from build123d import *

# Parameters (mm, degrees)
F0_W          = 105.2140146494
F0_H          = 74.0064755082
F0_R          = 22.3889711498
F1_DEPTH      = 22.86
F2_DEPTH      = 59.944
F3_DEPTH      = 25.4
F3_FACE_R     = 22.3889711498
F4_DEPTH      = 25.4
F4_TAPER      = -3
F5_DEPTH      = 25.4
F5_DEPTH_BACK = 25.4
F5_FACE_R     = 22.3889711498
F6_DEPTH      = 25.4
F6_TAPER      = -15
F7_DEPTH      = 59.182
F9_DEPTH      = 33.274


with BuildPart() as f1:
    # F0 (on Top) → F1 (new body)
    with BuildSketch(Plane.XY):
        Rectangle(F0_W, F0_H)
        Circle(F0_R, mode=Mode.SUBTRACT)
        Circle(F0_R)
    extrude(amount=F1_DEPTH)

    # F0 (on Top) → F2 (join)
    with BuildSketch(Plane.XY):
        Circle(F0_R)
    extrude(amount=F2_DEPTH)

    # F3 (cut): a face of the model
    f3_faces = [f1.faces().sort_by_distance(p)[0] for p in [
        (0, 0, 59.944),
    ]]
    extrude(f3_faces, amount=-F3_DEPTH, mode=Mode.SUBTRACT)

    # F3_face (on face) → F4 (join)
    with BuildSketch(Plane.XY.offset(34.544)):
        Circle(F3_FACE_R)
    extrude(amount=F4_DEPTH, taper=F4_TAPER)

    # F5 (cut, two sides): a face of the model
    f5_faces = [f1.faces().sort_by_distance(p)[0] for p in [
        (0, 0, 59.944),
    ]]
    extrude(f5_faces, amount=-F5_DEPTH, mode=Mode.SUBTRACT)
    extrude(f5_faces, amount=F5_DEPTH_BACK, mode=Mode.SUBTRACT)

    # F5_face (on face) → F6 (cut)
    with BuildSketch(Plane.XY.offset(34.544)):
        Circle(F5_FACE_R)
    extrude(amount=-F6_DEPTH, taper=F6_TAPER, mode=Mode.SUBTRACT)

    # F7 (add): a face of the model
    f7_faces = [f1.faces().sort_by_distance(p)[0] for p in [
        (0, 0, 9.144),
    ]]
    extrude(f7_faces, amount=F7_DEPTH)

    # F8 (on Front) → F9 (cut, symmetric)
    with BuildSketch(Plane.XZ):
        Polygon((-21.8193475157, 85.7371985912), (-29.5202936977, 68.7951147556), (38.5047309101, 34.6542596817), (50.8262440562, 89.5876735449), align=None)
    extrude(amount=F9_DEPTH, both=True, mode=Mode.SUBTRACT)


solid = f1.part
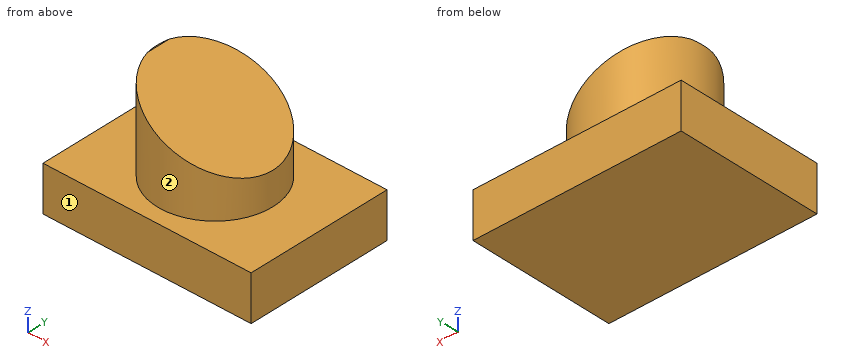
Geometry: final body of the model. Coordinates: model frame, mm. Face numbers are marked on the shaded views. A direction names the side the tool comes from. Coordinates: 2 decimals unless noted, no trailing zeros. Loops run counter-clockwise (first coordinate to the right, second up) from the corner with the lowest first, then second, coordinate; pieces in that order, holes last. Notation, with made-up numbers: (33.25, 3.25) - (89.25, 3.25) arc R32 ccw to (89.25, 40.25) - close; hole circle Ø8 at (8.25, 78). An arc over 180 degrees is marked (long way). One line per question, with ' | ' between items. Start each with the question number.
(1) Ray query, L1, parallel to Z at x = 30.5, y = -8; L2, parallel to X at y = 24, z = 46.5; L3, parallel to X at y = -15.5, z = 50.5. Return the intervals inside material, ascending. Write a range as from..to.
(2) Cut plane B-B on x = 4.5. Output: boundary loops of the cut face in (y, z), and give its area (3 significant figures).
(3) Cut plane A-A on y = 0. Output: boundary loops of the cut face in (x, z), and give its area (3 significant figures).
(4) First-contact query: pin 1 (6 mm diameter, centred on x = 7.5, z = 51.5, fed in from +Y); pin 2 (1.5 mm diameter, centred on x = -37, y = -29, fed in from +Z); pin 3 (10 mm diameter, centred on x = 16, z = 48.5, fed in from -Y). Flat tips, straight axial feed; report the tip coordinate or a pass-through.
(5) Cut plane C-C on z = 29. Output: boundary loops of the cut face in (x, y).
(6) Reachability of the marked faces 1 and 2 from +Z, -Z, +X, -X, +Y, -Y: full face, straight path, thin tool, end or side. Return the list, or none.
(7) Cut plane D-D on y = 9.5. Output: boundary loops of the cut face in (x, z).
Here are the results:
1) L1: 0..22.86 | L2: -16.62..14.9 | L3: -24.74..6.93
2) outline: (-37, 0) - (37, 0) - (37, 22.86) - (28.85, 22.86) - (28.85, 51.72) - (-28.85, 51.72) - (-28.85, 22.86) - (-37, 22.86) - close | area: 3,360 mm²
3) outline: (-52.61, 0) - (52.61, 0) - (52.61, 22.86) - (29.19, 22.86) - (29.19, 39.33) - (-28.59, 68.33) - (-29.19, 68.33) - (-29.19, 22.86) - (-52.61, 22.86) - close | area: 4,220 mm²
4) pin 1: y = 28.85 | pin 2: z = 22.86 | pin 3: y = -27.04
5) outline: circle Ø58.39 at (0, 0)
6) face 1: +Z, -Z, +X, -X, -Y | face 2: +Z
7) outline: (-52.61, 0) - (52.61, 0) - (52.61, 22.86) - (27.61, 22.86) - (27.61, 40.12) - (-27.61, 67.83) - (-27.61, 22.86) - (-52.61, 22.86) - close
